```python
from build123d import *

# Parameters (mm, degrees)
SKETCH3_R          = 1.5
CUT_EXTRUDE1_DEPTH = 4
SKETCH4_R          = 2.1
CUT_EXTRUDE2_DEPTH = 10


with BuildPart() as part:
    # Sketch2 → Revolve1 (revolve)
    with BuildSketch(Plane(origin=(0, 0, 0), x_dir=(1, 0, 0), z_dir=(0, 1, 0))):
        Polygon((0, 0), (0, 12), (-2.7, 12), (-2.7, 20), (-19.2, 20), (-19.2, 21), (-20.7, 21), (-20.7, 17.652837292), (-20.7, 14.5), (-20.7, 8), (-15.7, 8), (-15.7, 6), (-14.7, 6), (-14.7, 0), align=None)
    revolve(axis=Axis((0, 0, 0), (-1, 0, 0)))

    # Sketch3 → Cut-Extrude1 (cut)
    with BuildSketch(Plane.ZY.offset(20.7)):
        with Locations((0, 16)):
            Circle(SKETCH3_R)
        with Locations((13.856406461, 7.904729806)):
            Circle(SKETCH3_R)
        with Locations((13.773900052, -8.142905292)):
            Circle(SKETCH3_R)
        with Locations((-0.165012817, -16.095270194)):
            Circle(SKETCH3_R)
        with Locations((-14.021419278, -8)):
            Circle(SKETCH3_R)
        with Locations((-13.938912869, 8.047635097)):
            Circle(SKETCH3_R)
    extrude(amount=-CUT_EXTRUDE1_DEPTH, mode=Mode.SUBTRACT)

    # Sketch4 → Cut-Extrude2 (cut)
    with BuildSketch(Plane(origin=(-2.7, 0, 0), x_dir=(0, 0, -1), z_dir=(1, 0, 0))):
        with Locations((0, 16)):
            Circle(SKETCH4_R)
        with Locations((13.856406461, 8)):
            Circle(SKETCH4_R)
        with Locations((13.856406461, -8)):
            Circle(SKETCH4_R)
        with Locations((0, -16)):
            Circle(SKETCH4_R)
        with Locations((-13.856406461, -8)):
            Circle(SKETCH4_R)
        with Locations((-13.856406461, 8)):
            Circle(SKETCH4_R)
    extrude(amount=-CUT_EXTRUDE2_DEPTH, mode=Mode.SUBTRACT)


solid = part.part
```
Geometry check sheet. Reference: the model listing, model coordinates, mm. A direction names the side the tool comes from. Give positions to 0.01 mm unless a question says otherwise; leave off trailing zeros. Order: outer loops, then holes, each group sorted by start corner. A loop starts at its lowest first (then second) coordinate and runs counter-clockwise, first axis right, second up. Notation, with made-up numbers: (2, 69) - (27, 69) arc R20 cw to (27, 85) - close; hole circle Ø9 at (-18, 86). An arc over 180 degrees is marked (long way). Answer in a Markdown table with one row per item. Add a question column.
Q1. Cross-section at B-B, the plane z = -4.5. Enter the section's corners in (x, y), then the cut area to 3 significant figures.
Q2. Cross-section at A-A, the plane x = -10. Enter the section's corners in (y, z), then the cut area to 3 significant figures.
Q3. Mould release check, pull along Z, two halves, no side actions. Record for faces 3 (the flat face through (0, 0, 0)), 4 (the flat face through (-16.7, 8, -14)), 5 (the cylindrical face through (-1.37, -0.53, 11.99)): pulls with the +Z half, pulls with the -Z half, needs draft (parallel to the pull), parting line crosses it, or undercut.
Q4. Material ranges on probe 1 along Y at (x, z) = (-10.25, 0); probe 2 along Z at (x, y) = (-19.25, -7); probe 3 along Y at (x, z) = (-7, 12.5), recorded low to high. Write a range as from..to.
Q5. Gauge pin test, flat ends, axial feed: pin 1 (4 mm diameter, centred on x = -10.5, y = 16.5, fed in from -Z) (3 decimals); pin 2 (4.5 mm diameter, centred on y = -7.5, z = 14.5, fed in from +X); pin 3 (1 mm diameter, centred on x = -9, z = -9.5, fed in from -Y). Record the tip position at first contact, or that the pin passes through.
Q6. Tool access check on faces 1 (the flat face through (-12.7, 8, 14)), 2 (the flat face through (-16.7, -16, 0)). Record the directions out of +Z, -Z, +X, -X, +Y, -Y that give a thin tool (end or side, any length) a straight path to the whole face; none if there is none.
Q7. Cross-section at D-D, the plane z = 17.5. Enter the section's corners in (x, y), then the cut area to 3 significant figures.
Check values:
| question | item | result |
|---|---|---|
| 1 | outline | (-20.7, -20.51) - (-19.2, -20.51) - (-19.2, -19.49) - (-2.7, -19.49) - (-2.7, -11.12) - (0, -11.12) - (0, 11.12) - (-2.7, 11.12) - (-2.7, 19.49) - (-19.2, 19.49) - (-19.2, 20.51) - (-20.7, 20.51) - (-20.7, 6.61) - (-15.7, 6.61) - (-15.7, 3.97) - (-14.7, 3.97) - (-14.7, -3.97) - (-15.7, -3.97) - (-15.7, -6.61) - (-20.7, -6.61) - close |
| 1 | area | 691 mm^2 |
| 2 | outline | circle Ø40 at (0, 0); hole circle Ø4.2 at (-16, 0); hole circle Ø4.2 at (-8, -13.86); hole circle Ø4.2 at (-8, 13.86); hole circle Ø4.2 at (8, -13.86); hole circle Ø4.2 at (8, 13.86); hole circle Ø4.2 at (16, 0) |
| 2 | area | 1,170 mm^2 |
| 3 | face 3 | needs draft |
| 3 | face 4 | undercut |
| 3 | face 5 | parting line crosses it |
| 4 | probe 1 | y = -20..-18.1, -13.9..13.9, 18.1..20 |
| 4 | probe 2 | z = -19.8..-15.14, -12.9..-3.87, 3.87..12.8, 14.75..19.8 |
| 4 | probe 3 | y = -15.61..-9.6, -6.4..6.4, 9.6..15.61 |
| 5 | pin 1 | stops at z = -13.775 |
| 5 | pin 2 | stops at x = -2.7 |
| 5 | pin 3 | stops at y = -17.86 |
| 6 | face 1 | +X |
| 6 | face 2 | -X |
| 7 | outline | (-20.7, -11.61) - (-19.2, -11.61) - (-19.2, -9.68) - (-2.7, -9.68) - (-2.7, 9.68) - (-19.2, 9.68) - (-19.2, 11.61) - (-20.7, 11.61) - close |
| 7 | area | 354 mm^2 |
